Input: part model. Units: mm. Frame: model coordinates. Face numbers are marked on the shaded views. Round coordinates to 2 decimals unless told otherwise and drop trailing zeros. Loops run counter-clockwise (first coordinate to the right, second up) from the corner with the lowest first, then second, coordinate; pieces in that order, holes last. Notation, with made-up numbers: (78.25, -18.5) - (84.25, -18.5) arc R12 cw to (84.25, -2.5) - close; hole circle Ø3 at (32, 78.25). An arc over 180 degrees is marked (long way). Use CSV: the item, a comma, the result in double quotes. Start each with the question number.
1. Cut plane B-B (y = 0). Return loops of the section in (x, z), and give its area (3 significant figures).
2. Material intervals for probe 1 along Z at (x, y) = (33.5, -30.6); probe 2 along Z at (x, y) = (23.5, -6); probe 3 along X at (y, z) = (-23, -65.5), sorted ascending. Write a range as from..to.
3. Cut plane D-D (y = -28.5). Return loops of the section in (x, z), and give its area (3 significant figures).
4. Cut plane A-A (x = -33.5). Return loops of the section in (y, z).
5. Cut plane C-C (z = -64). Return loops of the section in (x, y).
6. Pin query (flat end, axial travel): P1, Ø5, axis at x = -22, z = -50, coming from the +Y side; P2, Ø1.5, axis at x = 12, z = -33, coming from the -Y side; P3, Ø7.5, axis at x = -27, z = -4.5, coming from the -Y side. Return the tip coordinate at first contact, or that it passes through.
7. Pull-direction query (X, two-part tool) for the marked faces 1 and 2; classes: +X half, -X half, draft (parallel to the pull), parting line (faces both ways), or undercut.
```python
from build123d import *

# Parameters (mm, degrees)
SKETCH_1_W          = 85
SKETCH_1_H          = 15
EXTRUDE_1_DEPTH     = 5
SKETCH_2_R          = 2.5
CUT_EXTRUDE_1_DEPTH = 5
SKETCH_3_W          = 45
SKETCH_3_H          = 6
EXTRUDE_2_DEPTH     = 67
SKETCH_4_W          = 45
SKETCH_4_H          = 6
EXTRUDE_3_DEPTH     = 30
SKETCH_7_W          = 20
SKETCH_7_H          = 15
EXTRUDE_4_DEPTH     = 6
CUT_EXTRUDE_3_DEPTH = 6
EXTRUDE_5_DEPTH     = 3
EXTRUDE_6_DEPTH     = 3
FILLET_1_R          = 1
SKETCH_11_R         = 2.5
CUT_EXTRUDE_4_DEPTH = 6
FILLET_2_R          = 1.5
EXTRUDE_7_DEPTH     = 2
EXTRUDE_8_DEPTH     = 2
EXTRUDE_9_DEPTH     = 3
EXTRUDE_10_DEPTH    = 3


with BuildPart() as part:
    # 草图1 → 凸台-拉伸1 (new body)
    with BuildSketch(Plane.XY):
        Rectangle(SKETCH_1_W, SKETCH_1_H)
    extrude(amount=EXTRUDE_1_DEPTH)

    # 草图2 → 切除-拉伸1 (cut)
    with BuildSketch(Plane.XY.offset(5)):
        with Locations((-37.5, 0)):
            Circle(SKETCH_2_R)
        with Locations((37.5, 0)):
            Circle(SKETCH_2_R)
    extrude(amount=-CUT_EXTRUDE_1_DEPTH, mode=Mode.SUBTRACT)

    # 草图3 → 凸台-拉伸2 (add)
    with BuildSketch(Plane(origin=(0, 0, 0), x_dir=(-1, 0, 0), z_dir=(0, 0, -1))):
        Rectangle(SKETCH_3_W, SKETCH_3_H)
    extrude(amount=EXTRUDE_2_DEPTH)

    # 草图4 → 凸台-拉伸3 (add)
    with BuildSketch(Plane.XZ.offset(3)):
        with Locations((0, -64)):
            Rectangle(SKETCH_4_W, SKETCH_4_H)
    extrude(amount=EXTRUDE_3_DEPTH)

    # 草图7 → 凸台-拉伸4 (add)
    with BuildSketch(Plane.XZ.offset(33)):
        with Locations((32.5, -64)):
            Rectangle(SKETCH_7_W, SKETCH_7_H)
        with Locations((-32.5, -64)):
            Rectangle(SKETCH_7_W, SKETCH_7_H)
    extrude(amount=-EXTRUDE_4_DEPTH)

    # 草图5 → 切除-拉伸3 (cut)
    with BuildSketch(Plane(origin=(0, 0, -67), x_dir=(-1, 0, 0), z_dir=(0, 0, -1))):
        with BuildLine():
            Line((-15.25, -33), (15.25, -33))
            ThreePointArc((15.25, -33), (0, -17.75), (-15.25, -33))
        make_face()
    extrude(amount=-CUT_EXTRUDE_3_DEPTH, mode=Mode.SUBTRACT)

    # 草图8 → 凸台-拉伸5 (add, symmetric)
    with BuildSketch(Plane(origin=(15, 0, 0), x_dir=(0, 0, -1), z_dir=(1, 0, 0))):
        Polygon((51, -3), (61, -13), (61, -3), align=None)
    extrude(amount=EXTRUDE_5_DEPTH, both=True)

    # 草图10 → 凸台-拉伸6 (add, symmetric)
    with BuildSketch(Plane(origin=(-15, 0, 0), x_dir=(0, 0, -1), z_dir=(1, 0, 0))):
        Polygon((61, -3), (51, -3), (61, -13), align=None)
    extrude(amount=EXTRUDE_6_DEPTH, both=True)

    # 圆角1
    fillet_1_edges = [part.edges().sort_by_distance(p)[0] for p in [
        (-20.25, -3, -61),
        (20.25, -3, -61),
        (0, -3, -61),
    ]]
    fillet(fillet_1_edges, radius=FILLET_1_R)

    # 草图11 → 切除-拉伸4 (cut)
    with BuildSketch(Plane.XZ.offset(33)):
        with Locations((-33.5, -64)):
            Circle(SKETCH_11_R)
        with Locations(Location((33.5, -64, 0), (0, 0, 180))):
            Circle(SKETCH_11_R)
    extrude(amount=-CUT_EXTRUDE_4_DEPTH, mode=Mode.SUBTRACT)

    # 圆角2
    # the kernel refuses this fillet: 1.5 mm, written as the material it adds along each edge
    with BuildSketch(Plane(origin=(-22.5, -27, -67), x_dir=(1, 0, 0), z_dir=(0, -1, 0)), Plane(origin=(22.5, -27, -61), x_dir=(-1, 0, 0), z_dir=(0, -1, 0)), Plane(origin=(22.5, -33, -67), x_dir=(-1, 0, 0), z_dir=(0, 1, 0))) as fillet_2_piece_1:
        with BuildLine():
            CenterArc((FILLET_2_R, -FILLET_2_R), FILLET_2_R, 90, 90)
            Line((0, -FILLET_2_R), (0, 0))
            Line((0, 0), (FILLET_2_R, 0))
        make_face()
    extrude(amount=6)
    with BuildSketch(Plane(origin=(-22.5, -27, -61), x_dir=(1, 0, 0), z_dir=(0, -1, 0))) as fillet_2_piece_2:
        with BuildLine():
            CenterArc((FILLET_2_R, FILLET_2_R), FILLET_2_R, 180, 90)
            Line((0, FILLET_2_R), (0, 0))
            Line((0, 0), (FILLET_2_R, 0))
        make_face()
    extrude(amount=6)

    # 草图12 → 凸台-拉伸7 (add, symmetric)
    with BuildSketch(Plane(origin=(0, 0, -64), x_dir=(-1, 0, 0), z_dir=(0, 0, -1))):
        Polygon((-22.5, -23), (-26.5, -27), (-22.5, -27), align=None)
    extrude_7 = extrude(amount=EXTRUDE_7_DEPTH, both=True)

    # 镜向1: 凸台-拉伸7 across plane
    add(extrude_7.mirror(Plane(origin=(0, 0, 0), x_dir=(0, 0, 1), z_dir=(1, 0, 0))))

    # 草图13 → 凸台-拉伸8 (add, symmetric)
    with BuildSketch(Plane(origin=(0, 0, 0), x_dir=(-1, 0, 0), z_dir=(0, -1, 0))):
        Polygon((-22.5, 7), (-29.5, 0), (-22.5, 0), align=None)
    extrude_8 = extrude(amount=EXTRUDE_8_DEPTH, both=True)

    # 镜向2: 凸台-拉伸8 across plane
    add(extrude_8.mirror(Plane(origin=(0, 0, 0), x_dir=(0, 0, 1), z_dir=(1, 0, 0))))

    # 草图14 → 凸台-拉伸9 (add, symmetric)
    with BuildSketch(Plane(origin=(15, 0, 0), x_dir=(0, 0, -1), z_dir=(1, 0, 0))):
        Polygon((0, 7.5), (8, 3), (0, 3), align=None)
        Polygon((8, -3), (0, -3), (0, -7.5), align=None)
    extrude(amount=EXTRUDE_9_DEPTH, both=True)

    # 草图15 → 凸台-拉伸10 (add, symmetric)
    with BuildSketch(Plane(origin=(-15, 0, 0), x_dir=(0, 0, -1), z_dir=(1, 0, 0))):
        Polygon((0, -7.5), (8, -3), (0, -3), align=None)
        Polygon((0, 7.5), (0, 3), (8, 3), align=None)
    extrude(amount=EXTRUDE_10_DEPTH, both=True)


solid = part.part
```
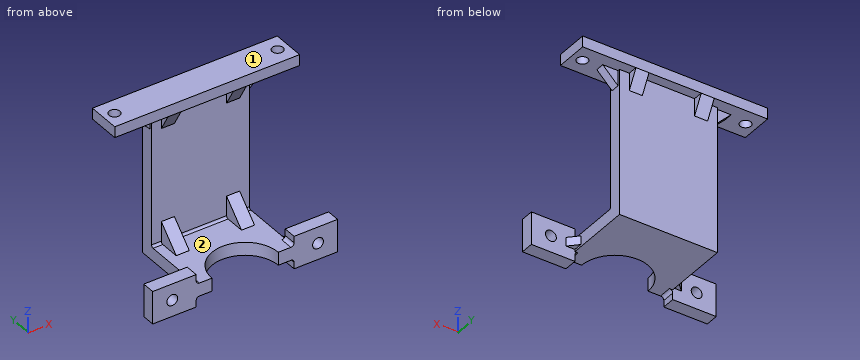
Established:
1,outline,"(-42.5, 0) - (-40, 0) - (-40, 5) - (-42.5, 5) - close; (-35, 0) - (-29.5, 0) - (-22.5, -7) - (-22.5, -67) - (22.5, -67) - (22.5, -7) - (29.5, 0) - (35, 0) - (35, 5) - (-35, 5) - close; (40, 0) - (42.5, 0) - (42.5, 5) - (40, 5) - close"
1,area,"3,440 mm2"
2,probe 1,"z = -71.5..-66.5, -61.5..-56.5"
2,probe 2,"z = 0..5"
2,probe 3,"x = -22.5..-11.51, 11.51..22.5"
3,outline,"(-42.5, -71.5) - (-22.5, -71.5) - (-22.5, -68.5) arc R1.5 cw to (-21, -67) - (-14.57, -67) - (-14.57, -61) - (-21, -61) arc R1.5 cw to (-22.5, -59.5) - (-22.5, -56.5) - (-42.5, -56.5) - close; (14.57, -67) - (21, -67) arc R1.5 cw to (22.5, -68.5) - (22.5, -71.5) - (42.5, -71.5) - (42.5, -56.5) - (22.5, -56.5) - (22.5, -59.5) arc R1.5 cw to (21, -61) - (14.57, -61) - close; hole circle Ø5 at (-33.5, -64); hole circle Ø5 at (33.5, -64)"
3,area,"658 mm2"
4,outline,"(-33, -71.5) - (-27, -71.5) - (-27, -66.5) - (-33, -66.5) - close; (-33, -61.5) - (-27, -61.5) - (-27, -56.5) - (-33, -56.5) - close; (-7.5, 0) - (7.5, 0) - (7.5, 5) - (-7.5, 5) - close"
5,outline,"(-42.5, -33) - (-36, -33) - (-36, -27) - (-42.5, -27) - close; (-31, -33) - (-15.25, -33) arc R15.25 cw to (15.25, -33) - (31, -33) - (31, -27) - (26.5, -27) - (22.5, -23) - (22.5, 3) - (-22.5, 3) - (-22.5, -23) - (-26.5, -27) - (-31, -27) - close; (36, -33) - (42.5, -33) - (42.5, -27) - (36, -27) - close"
6,P1,"stops at y = 3"
6,P2,"stops at y = -3"
6,P3,"stops at y = -2"
7,face 1,"draft"
7,face 2,"undercut"
